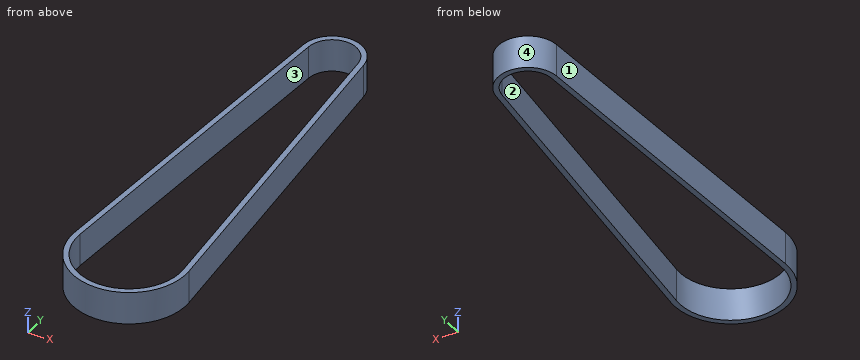
Autodesk Inventor part; units mm, degrees
ref_plane "YZ Plane" through (0, 0, 0) normal (1, 0, 0) x (0, 1, 0)
ref_plane "XZ Plane" through (0, 0, 0) normal (0, 1, 0) x (-1, 0, 0)
ref_plane "Work Plane1" through (0, 0, 1) normal (0, 0, 1) x (1, 0, 0)
sketch "Sketch1" plane through (0, 0, 1) normal (0, 0, 1) x (1, 0, 0)
  circle A0 centre (0, 0) radius 10.7044
  circle A1 centre (0.328, 62.3411) radius 5.7897
  arc A2 (5.8028, 62.7451) -> (-5.1423, 62.8026) centre (0.328, 62.3411) ccw
  arc A3 (-10.3676, 0.8748) -> (10.3762, 0.7656) centre (0, 0) ccw
  line L0 (-5.1423, 62.8026) -> (-10.3676, 0.8748)
  line L1 (5.8028, 62.7451) -> (10.3762, 0.7656)
  arc A4 (-5.1423, 62.8026) -> (5.8028, 62.7451) centre (0.328, 62.3411) ccw construction
  arc A5 (10.3762, 0.7656) -> (-10.3676, 0.8748) centre (0, 0) ccw construction
  line L2 (-9.3711, 0.7907) -> (-4.1458, 62.7186)
  arc A6 (4.8055, 62.6715) -> (-4.1458, 62.7186) centre (0.328, 62.3411) ccw
  line L3 (4.8055, 62.6715) -> (9.3789, 0.6921)
  arc A7 (-9.3711, 0.7907) -> (9.3789, 0.6921) centre (0, 0) ccw
  point P0 (0, 0)
  dimension "d1" = 0.3
  dimension "d2" = 0.3
  dimension "d3" = 1
extrude "Extrusion1" add sketch "Sketch1" along normal blind 6 contours L1 A3 L0 A0 L2 A7 L3 | A0 L3 A1 L1 | L0 A1 L2 A0 | A1 L3 A6 L2 L0 A2 L1
properties part number "Belt" material "Rubber"
Source: CAD feature listing. Evaluate the final solid. Frame: model axes, mm. Face numbers are marked on the shaded views. A direction names the side the tool comes from. Round coordinates to 2 decimals unless told otherwise and drop trailing zeros. Loops run counter-clockwise (first coordinate to the right, second up) from the corner with the lowest first, then second, coordinate; pieces in that order, holes last. Notation, with made-up numbers: (71.5, 89.25) -> (121.5, 89.25) arc R32 ccw to (121.5, 117.25) -> close; hole circle Ø10 at (87.25, 29). An arc over 180 degrees is marked (long way). Answer as a JSON object with one key per item and string values. Group by question number.
Q1. Section query A-A (z = 5.1). Output: boundary loops of the cut face in (x, y), plus the area to 3 significant figures.
Q2. Mould query, pull axis Y, two halves, no side actions, for the marked faces 1 and 2. Classes: pulls with the +Y half, pulls with the -Y half, needs draft (parallel to the pull), parting line crosses it, or undercut.
Q3. Contact query for flat-ended pins moving along their axis: P1, Ø3, axis at x = -3.5, y = 38, coming from the -Z side; P2, Ø2, axis at y = 16, z = 4, coming from the -X side; P3, Ø1, axis at x = -6.5, z = 5, coming from the -Y side. Output: stop coordinate, or through.
Q4. Section query C-C (y = -5). Output: boundary loops of the cut face in (x, z).
Q5. Access query for the marked faces 3 and 4. Directions: +Z, -Z, +X, -X, +Y, -Y. A direction counts if a zero-diameter tool reaches every point of the face in a straight line with its end or side. Return the directions, or none.
Q6. Section query B-B (x = -1). Output: boundary loops of the cut face in (y, z), plus the area to 3 significant figures.
Q7. Ray query, line 1 (X direction, y = 0, z = 6.75); line 2 (Y direction, x = 0.5, z = 1.7); line 3 (X direction, y = -2.5, z = 5). Return the intervals inside material, ascending. Write a range as from..to.
Completed:
{
 "1": {"outline": "(-10.37, 0.87) arc R10.4 ccw (long way) to (10.38, 0.77) -> (5.8, 62.75) arc R5.49 ccw to (-5.14, 62.8) -> close; hole (-9.37, 0.79) arc R9.4 ccw (long way) to (9.38, 0.69) -> (4.81, 62.67) arc R4.49 ccw to (-4.15, 62.72) -> close", "area": "172 mm²"},
 "2": {"face 1": "pulls with the +Y half", "face 2": "undercut"},
 "3": {"P1": "through", "P2": "x = -9.18", "P3": "y = -8.5"},
 "4": {"outline": "(-9.12, 1) -> (-7.97, 1) -> (-7.97, 7) -> (-9.12, 7) -> close; (7.97, 1) -> (9.12, 1) -> (9.12, 7) -> (7.97, 7) -> close"},
 "5": {"face 3": "+Z, -Z", "face 4": "+Z, -Z, +Y"},
 "6": {"outline": "(-10.36, 1) -> (-9.35, 1) -> (-9.35, 7) -> (-10.36, 7) -> close; (66.63, 1) -> (67.67, 1) -> (67.67, 7) -> (66.63, 7) -> close", "area": "12.3 mm²"},
 "7": {"line 1": "-10.4..-9.4, 9.4..10.4", "line 2": "-10.39..-9.39, 66.83..67.83", "line 3": "-10.1..-9.07, 9.07..10.1"}
}
